Geometry: final body of the model. Coordinates: model frame, mm. A direction names the side the tool comes from. Give positions to 0.01 mm unless a question says otherwise; leave off trailing zeros. Order: outer loops, then holes, each group sorted by start corner. A loop starts at its lowest first (then second) coordinate and runs counter-clockwise, first axis right, second up. Notation, with made-up numbers: (-20.75, 4.25) -> (16.25, 4.25) arc R9 cw to (16.25, 10.25) -> close; hole circle Ø11 at (-19, 6). An arc over 180 degrees is marked (long way). Answer in a Markdown table with one row per item. Add a question column.
Q1. Cut plane C-C on z = 38. Return the cut outline in (x, y), and give its area (3 significant figures).
Q2. Cut plane D-D on z = 12. Return the cut outline in (x, y), and give its area (4 significant figures).
Q3. Line query: line 1 along Y through (x, z) = (8, 33) (3 decimals); line 2 along Y through (x, z) = (-6, -10); line 3 along Y through (x, z) = (9, -6). Output: solid intervals per line, ascending. Write a range as from..to.
Q4. Contact query for flat-ended pins moving along their axis: P1, Ø1.5, axis at x = 8.5, y = 8, coming from the +Z side; P2, Ø1.8, axis at x = 1.875, z = 15, coming from the +Y side; P3, Ø10, axis at y = 15.5, z = 27, coming from the -X side; P4, Ø1.1, axis at y = 37.5, z = -5.5, coming from the +X side. Output: stop coordinate, or through.
Q5. Cut plane B-B on x = 2.5. Return the cut outline in (y, z) (3 decimals), and give its area (3 significant figures).
Q6. Set-up query: faces 5 (the face through (26.4, 44.9, -11.478)), 6 (the face through (15, -5.75, -7.7)), 7 (the face through (0.708, 36.603, -1.232)), 8 (the face through (-4, -2, 23)). Return all of +Z, -Z, +X, -X, +Y, -Y with unobstructed straight access to the full face (end or side cutting, diameter ignored); none if empty.
Q7. Pull-direction query (Y, two-part tool) for faces 1 (the face through (1.507, 29.33, -6.987)), 2 (the face through (11.512, -2.034, 40.743)), 3 (the face through (15.6, 0, -7.8)), 4 (the face through (15, -3, -8)); classes: +Y half, -Y half, draft (parallel to the pull), parting line (faces both ways), or undercut.
Q8. Cut plane A-A on y = 13.5. Return the cut outline in (x, z) (3 decimals).
from build123d import *

# Parameters (mm, degrees)
BOSS_EXTRUDE1_DEPTH = 21
BOSS_EXTRUDE2_DEPTH = 5.75
BOSS_EXTRUDE3_DEPTH = 7
SKETCH6_W           = 14.25
SKETCH6_H           = 13
BOSS_EXTRUDE4_DEPTH = 12
BOSS_EXTRUDE5_DEPTH = 29
SKETCH8_R           = 11.25
CUT_EXTRUDE1_DEPTH  = 2.5
SKETCH9_R           = 1.75
SKETCH9_R_2         = 7.5
CUT_EXTRUDE2_DEPTH  = 15.25
SKETCH10_W          = 30
SKETCH10_H          = 20.75
BOSS_EXTRUDE6_DEPTH = 23
CUT_EXTRUDE4_DEPTH  = 15
SKETCH12_W          = 37.5
SKETCH12_H          = 20.75
BOSS_EXTRUDE7_DEPTH = 20
SKETCH13_R          = 7.75
CUT_EXTRUDE5_DEPTH  = 43
SKETCH14_R          = 1.5
CUT_EXTRUDE6_DEPTH  = 10
CHAMFER1_SIZE       = 1


with BuildPart() as part:
    # Sketch1 → Boss-Extrude1 (new body)
    with BuildSketch(Plane(origin=(0, 0, 0), x_dir=(1, 0, 0), z_dir=(0, 1, 0))):
        with BuildLine():
            Line((23.125, 14.25), (30, 14.25))
            Line((30, 14.25), (30, 0))
            Line((30, 0), (0, 0))
            Line((0, 0), (0, 14.25))
            Line((0, 14.25), (6.875, 14.25))
            ThreePointArc((6.875, 14.25), (15, 6.125), (23.125, 14.25))
        make_face()
    extrude(amount=BOSS_EXTRUDE1_DEPTH)

    # Sketch2 → Boss-Extrude2 (add)
    with BuildSketch(Plane.XZ):
        with BuildLine():
            Line((21.25, -14.25), (30, -14.25))
            Line((30, -14.25), (30, 0))
            Line((30, 0), (0, 0))
            Line((0, 0), (0, -14.25))
            Line((0, -14.25), (8.75, -14.25))
            ThreePointArc((8.75, -14.25), (15, -8), (21.25, -14.25))
        make_face()
    extrude(amount=BOSS_EXTRUDE2_DEPTH)

    # Sketch3 → Boss-Extrude3 (add)
    with BuildSketch(Plane.XZ.offset(5.75)):
        with BuildLine():
            Line((23.25, -14.25), (30, -14.25))
            Line((30, -14.25), (30, 0))
            Line((30, 0), (0, 0))
            Line((0, 0), (0, -14.25))
            Line((0, -14.25), (6.75, -14.25))
            ThreePointArc((6.75, -14.25), (15, -6), (23.25, -14.25))
        make_face()
    extrude(amount=BOSS_EXTRUDE3_DEPTH)

    # Sketch6 → Boss-Extrude4 (add)
    with BuildSketch(Plane.ZY):
        with Locations((-7.125, 14.5)):
            Rectangle(SKETCH6_W, SKETCH6_H)
    extrude(amount=BOSS_EXTRUDE4_DEPTH)

    # Sketch7 → Boss-Extrude5 (add)
    with BuildSketch(Plane(origin=(0, 21, 0), x_dir=(1, 0, 0), z_dir=(0, 1, 0))):
        with BuildLine():
            Line((-12, 0), (30, 0))
            Line((30, 0), (30, 5.621629424))
            Line((30, 5.621629424), (30, 11.47775747))
            Line((30, 11.47775747), (24.530058266, 11.47775747))
            Line((24.530058266, 11.47775747), (22.637427339, 11.47775747))
            ThreePointArc((22.637427339, 11.47775747), (13.592603845, 6.24782148), (6.875, 14.25))
            Line((6.875, 14.25), (0.717619185, 14.25))
            Line((0.717619185, 14.25), (-12, 14.25))
            Line((-12, 14.25), (-12, 5.621629424))
            Line((-12, 5.621629424), (-12, 0))
        make_face()
    extrude(amount=BOSS_EXTRUDE5_DEPTH)

    # Sketch8 → Cut-Extrude1 (cut)
    with BuildSketch(Plane.XY):
        with Locations((9, 29)):
            Circle(SKETCH8_R)
    extrude(amount=-CUT_EXTRUDE1_DEPTH, mode=Mode.SUBTRACT)

    # Sketch9 → Cut-Extrude2 (cut, through all)
    with BuildSketch(Plane.XY):
        with Locations((-6.5, 44.5)):
            Circle(SKETCH9_R)
        with Locations((-6.5, 13.5)):
            Circle(SKETCH9_R)
        with Locations((24.5, 13.5)):
            Circle(SKETCH9_R)
        with Locations((24.5, 44.5)):
            Circle(SKETCH9_R)
        with Locations((9, 29)):
            Circle(SKETCH9_R_2)
    extrude(amount=-CUT_EXTRUDE2_DEPTH, mode=Mode.SUBTRACT)

    # Sketch10 → Boss-Extrude6 (add)
    with BuildSketch(Plane.XY):
        with Locations((15, -2.375)):
            Rectangle(SKETCH10_W, SKETCH10_H)
    extrude(amount=BOSS_EXTRUDE6_DEPTH)

    # Sketch11 → Cut-Extrude4 (cut)
    with BuildSketch(Plane(origin=(30, 0, 0), x_dir=(0, 0, -1), z_dir=(1, 0, 0))):
        Polygon((11.47775747, 17.5), (4, 17.5), (4, 40), (11.47775747, 40), (11.47775747, 21), (14.25, 21), (14.25, 17.5), align=None)
    extrude(amount=-CUT_EXTRUDE4_DEPTH, mode=Mode.SUBTRACT)

    # Sketch12 → Boss-Extrude7 (add)
    with BuildSketch(Plane.XY.offset(23)):
        with Locations((11.25, -2.375)):
            Rectangle(SKETCH12_W, SKETCH12_H)
    extrude(amount=BOSS_EXTRUDE7_DEPTH)

    # Sketch13 → Cut-Extrude5 (cut, through all)
    with BuildSketch(Plane(origin=(30, 0, 0), x_dir=(0, 0, -1), z_dir=(1, 0, 0))):
        with BuildLine():
            ThreePointArc((-43, 0.389168048), (-39.283405983, 5.880872713), (-33, 8))
            Line((-33, 8), (-43, 8))
            Line((-43, 8), (-43, 0.389168048))
        make_face()
        with BuildLine():
            ThreePointArc((-33, -12.75), (-39.283405983, -10.630872713), (-43, -5.139168048))
            Line((-43, -5.139168048), (-43, -12.75))
            Line((-43, -12.75), (-33, -12.75))
        make_face()
        with Locations((-33, -2.375)):
            Circle(SKETCH13_R)
    extrude(amount=-CUT_EXTRUDE5_DEPTH, mode=Mode.SUBTRACT)

    # Sketch14 → Cut-Extrude6 (cut)
    with BuildSketch(Plane(origin=(0, -12.75, 0), x_dir=(-1, 0, 0), z_dir=(0, -1, 0))):
        with Locations((-20.625, -15)):
            Circle(SKETCH14_R)
        with Locations((-1.875, -15)):
            Circle(SKETCH14_R)
    extrude(amount=-CUT_EXTRUDE6_DEPTH, mode=Mode.SUBTRACT)

    # Chamfer1
    chamfer1_edges = [part.edges().sort_by_distance(p)[0] for p in [
        (30, 29, 0),
        (30, 17.5, -9.125),
        (30, 40, -7.738878735),
        (30, 28.75, -4),
        (-12, 29, 0),
        (-12, 8, -7.125),
        (-12, 50, -7.125),
        (13.592603845, 50, -6.24782148),
        (30, 50, -5.738878735),
        (9, 50, 0),
    ]]
    chamfer(chamfer1_edges, length=CHAMFER1_SIZE)


solid = part.part
Completed:
| question | item | result |
|---|---|---|
| 1 | outline | (-7.5, -11.47) -> (30, -11.47) -> (30, -8.3) -> (-7.5, -8.3) -> close; (-7.5, 3.55) -> (30, 3.55) -> (30, 6.72) -> (-7.5, 6.72) -> close |
| 1 | area | 238 mm² |
| 2 | outline | (0, -12.75) -> (30, -12.75) -> (30, 8) -> (0, 8) -> close |
| 2 | area | 622.5 mm² |
| 3 | line 1 | y = -12.75..-10.125, 5.375..8 |
| 3 | line 2 | y = 8..11.82, 15.18..42.82, 46.18..50 |
| 3 | line 3 | y = -12.75..21.5, 36.5..50 |
| 4 | P1 | stops at z = 36.87 |
| 4 | P2 | stops at y = 8 |
| 4 | P3 | passes through |
| 4 | P4 | stops at x = 15 |
| 5 | outline | (-12.75, -14.25) -> (25.258, -14.25) -> (25.258, -2.5) -> (19.818, -2.5) -> (19.818, 0) -> (8, 0) -> (8, 33) arc R10.375 ccw to (0.389, 43) -> (-5.139, 43) arc R10.375 ccw to (-12.75, 33) -> (-12.75, 16.364) -> (-2.75, 16.364) -> (-2.75, 13.636) -> (-12.75, 13.636) -> close; (32.742, -14.25) -> (50, -14.25) -> (50, -1) -> (49, 0) -> (38.182, 0) -> (38.182, -2.5) -> (32.742, -2.5) -> close; hole circle Ø15.5 at (-2.375, 33) |
| 5 | area | 1,400 mm² |
| 6 | face 5 | -Z, +X, +Y |
| 6 | face 6 | -Z, -Y |
| 6 | face 7 | +Z |
| 6 | face 8 | -Z, -X, +Y, -Y |
| 7 | face 1 | undercut |
| 7 | face 2 | undercut |
| 7 | face 3 | +Y half |
| 7 | face 4 | draft |
| 8 | outline | (-12, -14.25) -> (-8.25, -14.25) -> (-8.25, 0) -> (-11, 0) -> (-12, -1) -> close; (-4.75, -14.25) -> (6.875, -14.25) arc R8.125 cw to (22.75, -11.81) -> (22.75, 0) -> (-4.75, 0) -> close; (26.25, -14.25) -> (30, -14.25) -> (30, -1) -> (29, 0) -> (26.25, 0) -> close |
